CAD build for the part. Positions are in the model's coordinates, mm. A direction names the side the tool comes from. Give positions to 0.01 mm unless a question says otherwise; leave off trailing zeros. Loops run counter-clockwise (first coordinate to the right, second up) from the corner with the lowest first, then second, coordinate; pieces in that order, holes last. Notation, with made-up numbers: (73, -23.75) - (109, -23.75) arc R19 ccw to (109, 5.25) - close; hole circle Ø7 at (57.5, -33.75). An arc over 180 degrees is marked (long way). Return JSON: item names as keys, results as strings.
from build123d import *

# Parameters (mm, degrees)
ESBO_O1_W                  = 77
ESBO_O1_H                  = 5
RESSALTO_EXTRUS_O1_DEPTH   = 5
ESBO_O2_W                  = 2
ESBO_O2_H                  = 50
RESSALTO_EXTRUS_O2_DEPTH   = 5
FILETE1_R                  = 2.5
ESBO_O7_R                  = 2.5
RESSALTO_EXTRUS_O5_DEPTH   = 5
ESBO_O3_R                  = 1
CORTE_EXTRUS_O1_DEPTH      = 62.347371582
FILETE1_OF_ESPELHAR1_R     = 2.5
FILETE2_R                  = 2.5
ESBO_O4_W                  = 30
ESBO_O4_H                  = 5
RESSALTO_EXTRUS_O3_DEPTH   = 1
FILETE3_R                  = 2.5
ESBO_O6_R                  = 2.5
RESSALTO_EXTRUS_O4_DEPTH   = 5
CORTE_EXTRUS_O2_DEPTH      = 62.347371582
CORTE_EXTRUS_O2_DEPTH_BACK = 62.347371582
ESBO_O5_R                  = 1


with BuildPart() as part:
    # Esboço1 → Ressalto-extrusão1 (new body)
    with BuildSketch(Plane(origin=(0, 0, 0), x_dir=(1, 0, 0), z_dir=(0, 1, 0))):
        Rectangle(ESBO_O1_W, ESBO_O1_H)
    extrude(amount=RESSALTO_EXTRUS_O1_DEPTH)

    # Esboço2 → Ressalto-extrusão2 (add)
    with BuildSketch(Plane(origin=(0, 0, 0), x_dir=(1, 0, 0), z_dir=(0, 1, 0))):
        with Locations((-37.5, -22.5)):
            Rectangle(ESBO_O2_W, ESBO_O2_H)
    ressalto_extrus_o2 = extrude(amount=RESSALTO_EXTRUS_O2_DEPTH)

    # Filete1
    filete1_edges = [part.edges().sort_by_distance(p)[0] for p in [
        (-37.5, 0, 47.5),
        (-37.5, 5, 47.5),
    ]]
    fillet(filete1_edges, radius=FILETE1_R - 0.0001)  # a hair under: the kernel refuses the full size

    # Esboço7 → Ressalto-extrusão5 (add)
    with BuildSketch(Plane(origin=(-36.5, 0, 0), x_dir=(0, 0, -1), z_dir=(1, 0, 0))):
        with Locations((-45, 2.5)):
            Circle(ESBO_O7_R)
    ressalto_extrus_o5 = extrude(amount=RESSALTO_EXTRUS_O5_DEPTH)

    # Esboço3 → Corte-extrusão1 (cut, through all)
    with BuildSketch(Plane(origin=(0, 0, 0), x_dir=(0, 0, -1), z_dir=(1, 0, 0))):
        with Locations((-45, 2.5)):
            Circle(ESBO_O3_R)
    corte_extrus_o1 = extrude(amount=-CORTE_EXTRUS_O1_DEPTH, mode=Mode.SUBTRACT)

    # Espelhar1: Ressalto-extrusão2, Ressalto-extrusão5, Corte-extrusão1 across plane
    add(ressalto_extrus_o2.mirror(Plane(origin=(0, 0, 0), x_dir=(0, 0, 1), z_dir=(1, 0, 0))))
    add(ressalto_extrus_o5.mirror(Plane(origin=(0, 0, 0), x_dir=(0, 0, 1), z_dir=(1, 0, 0))))
    add(corte_extrus_o1.mirror(Plane(origin=(0, 0, 0), x_dir=(0, 0, 1), z_dir=(1, 0, 0))), mode=Mode.SUBTRACT)

    # Filete1 of Espelhar1
    filete1_of_espelhar1_edges = [part.edges().sort_by_distance(p)[0] for p in [
        (37.5, 0, 47.5),
        (37.5, 5, 47.5),
    ]]
    fillet(filete1_of_espelhar1_edges, radius=FILETE1_OF_ESPELHAR1_R - 0.0001)  # a hair under: the kernel refuses the full size

    # Filete2
    filete2_edges = [part.edges().sort_by_distance(p)[0] for p in [
        (-38.5, 2.5, -2.5),
        (38.5, 2.5, -2.5),
    ]]
    fillet(filete2_edges, radius=FILETE2_R)

    # Esboço4 → Ressalto-extrusão3 (add, symmetric)
    with BuildSketch(Plane(origin=(0, 0, 0), x_dir=(0, 0, -1), z_dir=(1, 0, 0))):
        with Locations((12.5, 2.5)):
            Rectangle(ESBO_O4_W, ESBO_O4_H)
    extrude(amount=RESSALTO_EXTRUS_O3_DEPTH, both=True)

    # Filete3
    filete3_edges = [part.edges().sort_by_distance(p)[0] for p in [
        (0, 5, -27.5),
        (0, 0, -27.5),
    ]]
    fillet(filete3_edges, radius=FILETE3_R - 0.0001)  # a hair under: the kernel refuses the full size

    # Esboço6 → Ressalto-extrusão4 (add)
    with BuildSketch(Plane.ZY.offset(1)):
        with Locations((-25, 2.5)):
            Circle(ESBO_O6_R)
    extrude(amount=RESSALTO_EXTRUS_O4_DEPTH)

    # Esboço5 → Corte-extrusão2 (cut, two sides: drawn at the far end of the back side and taken through both)
    with BuildSketch(Plane(origin=(0, 0, 0), x_dir=(0, 0, -1), z_dir=(1, 0, 0)).offset(-CORTE_EXTRUS_O2_DEPTH_BACK)):
        with Locations((25, 2.5)):
            Circle(ESBO_O5_R)
    extrude(amount=CORTE_EXTRUS_O2_DEPTH + CORTE_EXTRUS_O2_DEPTH_BACK, mode=Mode.SUBTRACT)


solid = part.part
1. Cut at A-A, the plane z = 15. Write the cut outline in (x, y).
Values follow:
{"outline": "(-38.5, 0) - (-36.5, 0) - (-36.5, 5) - (-38.5, 5) - close; (36.5, 0) - (38.5, 0) - (38.5, 5) - (36.5, 5) - close"}
2. Which spindle directions (+Z, -Z, +X, -X, +Y, -Y) get a long thin tool onto all of the face, cutting with end or side? Do faces 1 (the face through (1, 2, 2.5)), 2 (the face through (18, 2, -2.5)), 3 (the face through (-31.5, 1, 45)), 4 (the face through (-6, 1, -25)). Say none if no direction does.
Values follow:
{"face 1": "+Y, -Y", "face 2": "-Z, +X, +Y, -Y", "face 3": "+Z, +Y, -Y", "face 4": "-Z, -X, +Y, -Y"}
3. Drop flat-ended pins along their axis: P1, Ø2.5, axis at y = 3.5, z = -14.5, coming from the +X side; P2, Ø1.5, axis at x = 10.5, y = 2.5, coming from the +Z side. Give the stop position or say it passes through.
Values follow:
{"P1": "stops at x = 1", "P2": "stops at z = 2.5"}
4. Pull direction X, two halves, no side cores. Call faces 5 (the face through (0, 4, -27)), 6 (the face through (-1, 3, -14)), 7 (the face through (31.5, 1, 45)): +X half, -X half, draft (parallel to the pull), parting line (faces both ways), or undercut.
Values follow:
{"face 5": "draft", "face 6": "-X half", "face 7": "undercut"}
5. Cut at C-C, the plane x = 28. Write the cut outline in (y, z).
Values follow:
{"outline": "(0, -2.5) - (5, -2.5) - (5, 2.5) - (0, 2.5) - close"}
6. Cut at D-D, the plane z = -16.5. Write the cut outline in (x, y).
Values follow:
{"outline": "(-1, 0) - (1, 0) - (1, 5) - (-1, 5) - close"}
7. Drill centre lines: probe 1 along Z at (x, y) = (-3, 2.5); probe 2 along Y at (x, z) = (-34, 45); probe 3 along Z at (x, y) = (32, 3). Where is each one in solid material? Low to high.
Values follow:
{"probe 1": "z = -27.5 to -26, -24 to -22.5, -2.5 to 2.5", "probe 2": "y = 0 to 1.5, 3.5 to 5", "probe 3": "z = -2.5 to 2.5, 42.55 to 44.13, 45.87 to 47.45"}
